Source: CAD feature listing. Evaluate the final solid. Frame: model axes, mm. A direction names the side the tool comes from. Coordinates: 2 decimals unless noted, no trailing zeros. Write each loop counter-clockwise with the first axis right and the second up, starting at its lowest first coordinate (ties: lowest second). Pieces come first, ordered by that corner, then holes. Notation, with made-up numbers: (86.25, 56.5) -> (140.25, 56.5) arc R25 cw to (140.25, 76.5) -> close; hole circle Ø11 at (48, -26). An arc over 180 degrees is marked (long way). Write item = value, one per line.
from build123d import *

# Parameters (mm, degrees)
BASEHEAD_DEPTH    = 6.8
FLANGEHEXFILLET_R = 0.11


with BuildPart() as part:
    # Sketch1 → BaseHead (new body)
    with BuildSketch(Plane(origin=(0, 0, 0), x_dir=(0, 0, -1), z_dir=(1, 0, 0))):
        Polygon((4, 2.309401077), (4, -2.309401077), (0, -4.618802154), (-4, -2.309401077), (-4, 2.309401077), (0, 4.618802154), align=None)
    extrude(amount=BASEHEAD_DEPTH)

    # BodySke → BaseBody (revolve)
    with BuildSketch(Plane.XY, mode=Mode.PRIVATE) as basebody_sk:
        Polygon((0, 0), (66.8, 0), (66.8, 2.4455), (66.2455, 3), (0, 3), align=None)
    revolve(basebody_sk.sketch.rotate(Axis((0, 0, 0), (1, 0, 0)), 90), axis=Axis((0, 0, 0), (1, 0, 0)))  # turned: the seam where the file's is

    # Sketch3 → HeadChamfer (revolve, cut)
    with BuildSketch(Plane.XY, mode=Mode.PRIVATE) as headchamfer_sk:
        Polygon((0, 4), (3.244016936, 9.618802154), (3.244016936, 14.618802154), (-10, 14.618802154), (-10, 4), align=None)
    revolve(headchamfer_sk.sketch.rotate(Axis((0, 0, 0), (1, 0, 0)), 90), axis=Axis((0, 0, 0), (1, 0, 0)), mode=Mode.SUBTRACT)  # turned: the seam where the file's is

    # Sketch4 → Flange (revolve)
    with BuildSketch(Plane.XY, mode=Mode.PRIVATE) as flange_sk:
        with BuildLine():
            Line((3.389888261, 0), (5.733169059, 6.438111079))
            ThreePointArc((5.733169059, 6.438111079), (6.345506498, 6.791644264), (6.8, 6.25))
            Line((6.8, 6.25), (6.8, 0))
            Line((6.8, 0), (3.389888261, 0))
        make_face()
    revolve(flange_sk.sketch.rotate(Axis((0, 0, 0), (1, 0, 0)), 90), axis=Axis((0, 0, 0), (1, 0, 0)))  # turned: the seam where the file's is

    # FlangeHexFillet
    flangehexfillet_edges = [part.edges().sort_by_distance(p)[0] for p in [
        (4.845769198, 0, -4),
        (4.845769198, -3.464101615, -2),
        (4.905726696, 1.159737717, 4),
        (4.845769198, 3.464101615, 2),
        (4.845769198, 3.464101615, -2),
        (4.845769198, -3.464101615, 2),
        (4.905726696, -1.159737717, 4),
    ]]
    fillet(flangehexfillet_edges, radius=FLANGEHEXFILLET_R)


solid = part.part
1) Reachability of faces 1 (the flat face through (6.8, -3, -1)), 2 (the flat face through (2.459, 3.448, 2.028)), 3 (the flat face through (2.459, -3.448, -2.028)) from +Z, -Z, +X, -X, +Y, -Y: full face, straight path, thin tool, end or side. Return the list, or none.
Answer block:
face_1 = +X
face_2 = +Z, -X, +Y
face_3 = -Z, -X, -Y
2) Cut plane A-A, the plane x = 19. Output: boundary loops of the cut face in (y, z).
Answer block:
outline = circle Ø6 at (0, 0)
3) First-contact query: pin 1 Ø5 at (x, z) = (23, -3.5) entering from +Y; pin 2 Ø3 at (y, z) = (0, 4) entering from +X; pin 3 Ø1.5 at (x, y) = (54, -2) entering from +Z. Flat tips, straight axial feed; report the tip coordinate or a pass-through.
Answer block:
pin_1 = 2.83
pin_2 = 66.75
pin_3 = 2.73
4) Material intervals for probe 1 along X at (y, z) = (2.5, 3); probe 2 along Y at (x, z) = (21, -1.75); probe 3 along X at (y, z) = (-5, 2.5), sorted ascending. Write a range as [from, to].
Answer block:
probe_1 = [0, 6.8]
probe_2 = [-2.44, 2.44]
probe_3 = [5.42, 6.8]
